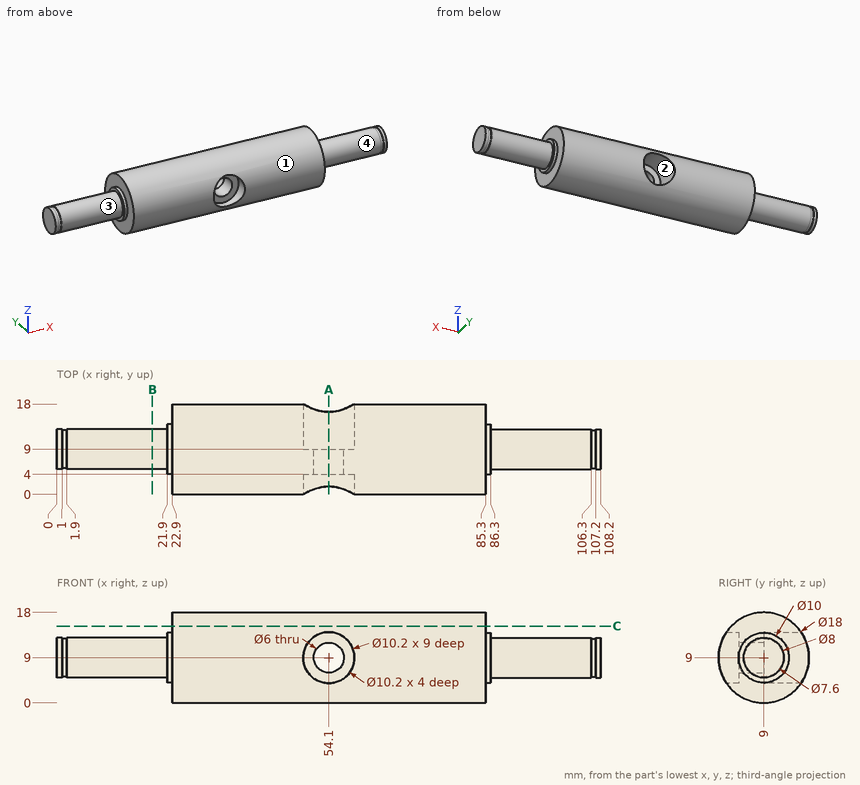
Design review of the part shown in the three views and the two pictorial views. Dimensions are in mm from the part's minimum x, y and z. A direction names the side the tool comes from. Round coordinates to 2 decimals unless told otherwise and drop trailing zeros. Loops run counter-clockwise (first coordinate to the right, second up) from the corner with the lowest first, then second, coordinate; pieces in that order, holes last. Notation, with made-up numbers: M 61.25,-31 L 101.25,-31 A23 ccw 101.25,-17 Z; hole C 80.25,25 d11. An arc over 180 degrees is marked long. Answer as a JSON object with one key per item and string values.
Item 1: Clearance check with flat-ended pins moving along their axes: P1, Ø9.5, axis at x = 54.1, z = 9, coming from the +Y side; P2, Ø9, axis at x = 54.1, z = 9, coming from the -Y side; P3, Ø4, axis at y = 9, z = 7.5, coming from the -X side; P4, Ø4, axis at x = 26, y = 16, coming from the +Z side. State where each tip first meets the part, or that it passes through.
Answer sheet:
{"P1": "stops at y = 9", "P2": "stops at y = 4", "P3": "stops at x = 0", "P4": "stops at z = 16.48"}
Item 2: The part is to be moulded in two halves that separate along Z. For the marked faces 1 and 2, say which applies: pulls with the +Z half, pulls with the -Z half, needs draft (parallel to the pull), parting line crosses it, or undercut.
Answer sheet:
{"face 1": "parting line crosses it", "face 2": "undercut"}
Item 3: We need section C-C on z = 15.25. Give the boundary of the cut face in (x, y).
Answer sheet:
{"outline": "M 22.9,2.52 L 85.3,2.52 L 85.3,15.48 L 22.9,15.48 Z"}
Item 4: Machinability: for the marked faces 3 and 4, which of the approach directions +Z, -Z, +X, -X, +Y, -Y give a long, thin tool a straight path to every point of the face, cutting with its end or side? Answer none if there is none.
Answer sheet:
{"face 3": "-X", "face 4": "+X"}
Item 5: Wall thickness on L1, parallel to X at y = 7.3, z = 9; L2, parallel to Z at x = 54.1, y = 2.5; L3, parallel to X at y = 7.5, z = 11: over which ranges is each line inside the solid? List them lowest first. Write a range as from..to.
Answer sheet:
{"L1": "x = 0..51.1, 57.1..108.2", "L2": "z = 2.78..3.9, 14.1..15.22", "L3": "x = 0..51.86, 56.34..108.2"}
Item 6: We need section A-A on x = 54.1. Give the boundary of the cut face in (y, z).
Answer sheet:
{"outline": "M 1.58,3.9 A9 ccw 16.42,3.9 L 9,3.9 L 9,6 L 4,6 L 4,3.9 Z; M 1.58,14.1 L 4,14.1 L 4,12 L 9,12 L 9,14.1 L 16.42,14.1 A9 ccw Z"}
Item 7: We need section B-B on x = 19. Give the boundary of the cut face in (y, z), and give its area (3 significant figures).
Answer sheet:
{"outline": "C 9,9 d8", "area": "50.3 mm^2"}
